Read the model definition and answer for the solid it produces. Units are mm, in the model's axes. Face numbers are marked on the shaded views. Coordinates: 2 decimals unless noted, no trailing zeros. Write each loop counter-clockwise with the first axis right and the second up, starting at its lowest first coordinate (ties: lowest second). Pieces come first, ordered by that corner, then holes.
(1) Given pin 1 (1.5 mm diameter, centred on x = 2, z = 7.5, fed in from -Y); pin 2 (2 mm diameter, centred on x = -2, z = 21, fed in from -Y); pin 3 (1.5 mm diameter, centred on x = 1.5, z = 19.5, fed in from +Y), each flat-ended and moving along its own axis, determine where each tip first touches the part or whether it passes through.
(2) Section C-C on x = 1.75 is taken. Write down the section's boundary in (y, z).
(3) Section B-B on x = -1.5 is taken. Write down the section's boundary in (y, z).
(4) Find the intervals of material crossed by probe 1 along Y at (x, z) = (-2.25, 13.75); probe 2 along Y at (x, z) = (1, 26), in increasing order.
(5) The mould has two halves that part along Z. Classify the marked faces 1, 2 and 3: +Z half, -Z half, draft (parallel to the pull), parting line (faces both ways), or undercut.
from build123d import *

# Parameters (mm, degrees)
F0_W     = 75
F0_H     = 30
F1_DEPTH = 3
F2_SIZE  = 2.99999


# Not quite as in the source:
# - a fillet or chamfer is up to 0.001 mm smaller than in the source, because OpenCascade refuses the exact size


with BuildPart() as f1:
    # F0 (on Right) → F1 (new body, symmetric)
    with BuildSketch(Plane.YZ):
        with Locations((0, 15)):
            Rectangle(F0_W, F0_H)
    extrude(amount=F1_DEPTH, both=True)

    # F2 (size 3 in the source; OpenCascade refuses exactly that, so slightly less here)
    f2_edges = [f1.edges().sort_by_distance(p)[0] for p in [
        (3, -37.5, 15),
        (-3, -37.5, 15),
        (-3, 37.5, 15),
        (3, 37.5, 15),
    ]]
    chamfer(f2_edges, length=F2_SIZE)


solid = f1.part
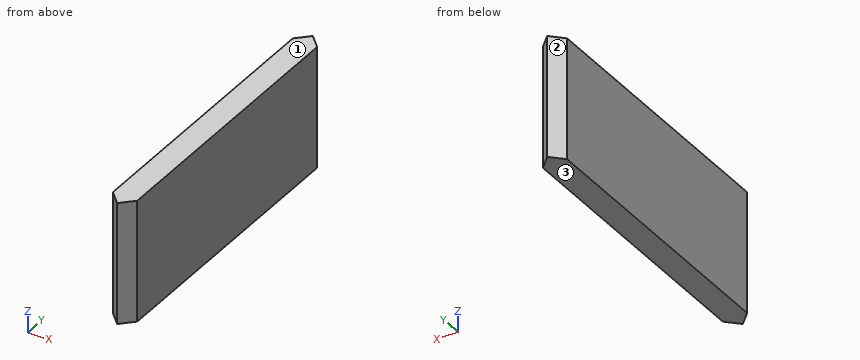
Response:
1. pin 1: stops at y = -36.25
1. pin 2: stops at y = -36.5
1. pin 3: stops at y = 36.75
2. outline: (-35.75, 0) - (35.75, 0) - (35.75, 30) - (-35.75, 30) - close
3. outline: (-36, 0) - (36, 0) - (36, 30) - (-36, 30) - close
4. probe 1: y = -35.25 to 35.25
4. probe 2: y = -36.5 to 36.5
5. face 1: +Z half
5. face 2: draft
5. face 3: -Z half
